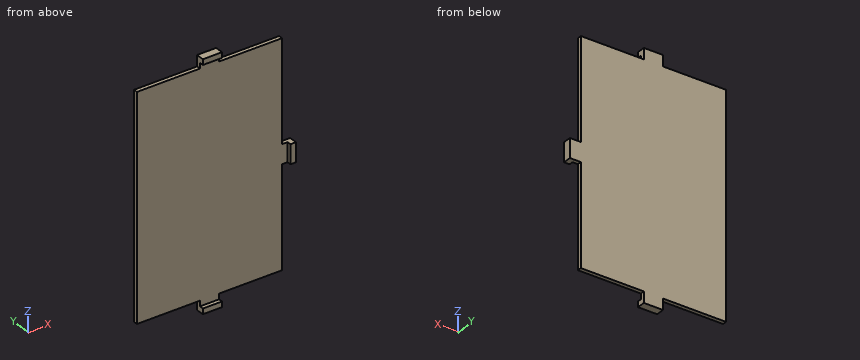
from build123d import *

# Parameters (mm, degrees)
BOSS_EXTRUDE1_DEPTH = 1.5
SKETCH2_W           = 7
SKETCH2_H           = 2
SKETCH2_W_2         = 2
SKETCH2_H_2         = 7
BOSS_EXTRUDE2_DEPTH = 3


with BuildPart() as part:
    # Sketch1 → Boss-Extrude1 (new body)
    with BuildSketch(Plane(origin=(0, 0, 0), x_dir=(1, 0, 0), z_dir=(0, 1, 0))):
        Polygon((30, 81), (53, 81), (53, 44), (55, 44), (55, 37), (53, 37), (53, 0), (30, 0), (30, -2), (23, -2), (23, 0), (0, 0), (0, 81), (23, 81), (23, 83), (30, 83), align=None)
    extrude(amount=BOSS_EXTRUDE1_DEPTH)

    # Sketch2 → Boss-Extrude2 (add)
    with BuildSketch(Plane(origin=(0, 1.5, 0), x_dir=(1, 0, 0), z_dir=(0, 1, 0))):
        with Locations((26.5, 84)):
            Rectangle(SKETCH2_W, SKETCH2_H)
        with Locations((56, 40.5)):
            Rectangle(SKETCH2_W_2, SKETCH2_H_2)
        with Locations((26.5, -3)):
            Rectangle(SKETCH2_W, SKETCH2_H)
    extrude(amount=-BOSS_EXTRUDE2_DEPTH)


solid = part.part
Here's how the part is built. I have some questions about the finished solid (model axes, mm). Coordinates: 2 decimals unless noted, no trailing zeros. Write each loop counter-clockwise with the first axis right and the second up, starting at its lowest first coordinate (ties: lowest second). Pieces come first, ordered by that corner, then holes.
1) I'm going to push flat-ended pins straight in: pin 1 (1.5 mm diameter, centred on y = -1, z = -46.5, fed in from -X); pin 2 (0.8 mm diameter, centred on y = 0.5, z = -19.5, fed in from +X); pin 3 (1.5 mm diameter, centred on x = 32.5, z = -8.5, fed in from -Y); pin 4 (1.5 mm diameter, centred on x = 55.5, y = -0.5, fed in from +Z). Where does each tip first touch, or does it pass through?
Filled in:
pin 1: passes through
pin 2: stops at x = 53
pin 3: stops at y = 0
pin 4: stops at z = -37
2) If we section it at C-C (z = -49.5): List the corners of the cut face in (x, y) for me, plus the area to 3 significant figures.
Filled in:
outline: (0, 0) - (53, 0) - (53, 1.5) - (0, 1.5) - close
area: 79.5 mm2
3) If we section it at A-A (y = -0.6): List the corners of the cut face in (x, z) for me.
Filled in:
outline: (23, -85) - (30, -85) - (30, -83) - (23, -83) - close; (23, 2) - (30, 2) - (30, 4) - (23, 4) - close; (55, -44) - (57, -44) - (57, -37) - (55, -37) - close
4) If we section it at B-B (x = 26): List the corners of the cut face in (y, z) for me, plus the area to 4 significant figures.
Filled in:
outline: (-1.5, -85) - (1.5, -85) - (1.5, 4) - (-1.5, 4) - (-1.5, 2) - (0, 2) - (0, -83) - (-1.5, -83) - close
area: 139.5 mm2
5) If I drill on line 1 (Y direction, x = 13, z = -75.5); line 2 (X direction, y = 0.15, z = -73); line 3 (Z direction, x = 49, y = 1.35), over which ranges is the centre line in solid material (lowest first)?
Filled in:
line 1: y = 0 to 1.5
line 2: x = 0 to 53
line 3: z = -81 to 0
6) If we section it at D-D (x = 39.5): List the corners of the cut face in (y, z) for me.
Filled in:
outline: (0, -81) - (1.5, -81) - (1.5, 0) - (0, 0) - close
